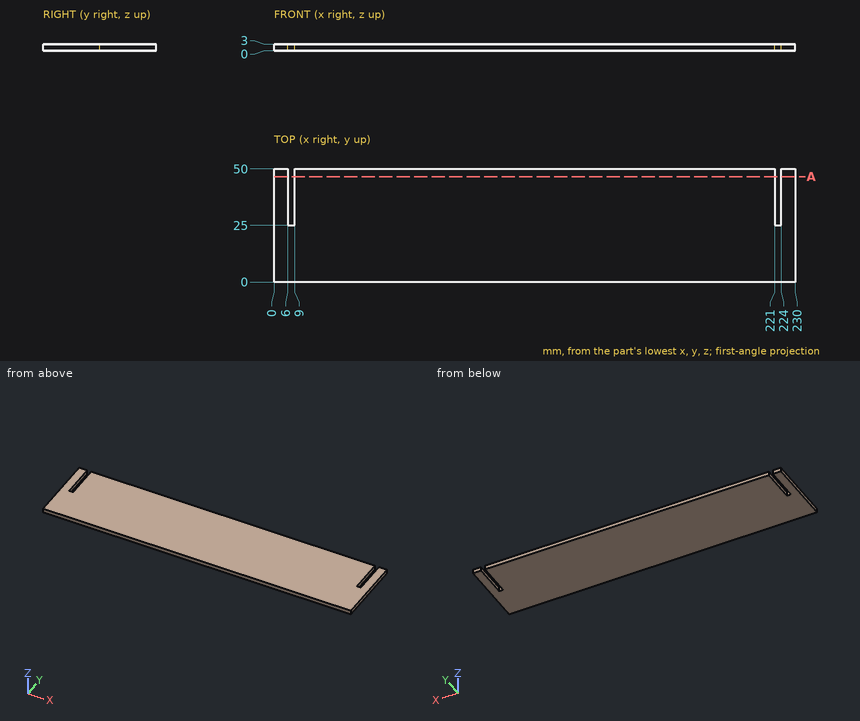
Drawing for the job (mm, zero at the part's lowest x, y, z). Round coordinates to 2 decimals unless told otherwise and drop trailing zeros. Write each loop counter-clockwise with the first axis right and the second up, starting at its lowest first coordinate (ties: lowest second). Pieces come first, ordered by that corner, then holes. Notation, with made-up numbers: (59.25, 36) - (96.25, 36) arc R25 ccw to (96.25, 64) - close; hole circle Ø5 at (-4.5, 23). An arc over 180 degrees is marked (long way). Write item = value, one per line. Start each with the question number.
Q1. Probe L1, parallel to X at y = 30, z = 0.85. List the from-to ranges inside material, lowest first. Write a range as from..to.
Q2. Drop flat-ended pins along their axis: pin 1 (5 mm diameter, centred on x = 158, y = 32, fed in from -Z); pin 2 (0.9 mm diameter, centred on x = 222, z = 1, fed in from +Y). Give the stop position or say it passes through.
Q3. Band-saw the part on A-A (y = 46.5). Give the cut face in (x, z), then the cut area to 3 significant figures.
Answers below:
q1.L1 = 0..6, 9..221, 224..230
q2.pin_1 = 0
q2.pin_2 = 25
q3.outline = (0, 0) - (6, 0) - (6, 3) - (0, 3) - close; (9, 0) - (221, 0) - (221, 3) - (9, 3) - close; (224, 0) - (230, 0) - (230, 3) - (224, 3) - close
q3.area = 672 mm2
